Here's how the part is built. I have some questions about the finished solid (model axes, mm). Round coordinates to 2 decimals unless told otherwise and drop trailing zeros. Order: outer loops, then holes, each group sorted by start corner. A loop starts at its lowest first (then second) coordinate and runs counter-clockwise, first axis right, second up. Notation, with made-up numbers: M 22.25,-23 L 44.25,-23 A25 cw 44.25,-11 Z; hole C 16.25,-38 d1. An arc over 180 degrees is marked long. Write item = value, one per line. Start each with the question number.
Item 1: I want a section at C-C, the plane z = -23.5. List the corners of the cut face in (x, y) for me, plus the area to 3 significant figures.
Item 2: I want a section at A-A, the plane x = 23.5. List the corners of the cut face in (y, z) for me, plus the area to 3 significant figures.
Item 3: I want a section at D-D, the plane x = 5. List the corners of the cut face in (y, z) for me, plus the area to 3 significant figures.
Item 4: I want a section at B-B, the plane z = -17.5. List the corners of the cut face in (x, y) for me.
Item 5: Please list where these lines run through material, in increasing order: L1, parallel to Z at x = -23.5, y = 1.1; L2, parallel to X at y = 1.5, z = -23.5; L3, parallel to X at y = 1.55, z = 23.5.
Item 6: I'm going to push flat-ended pins straight in: P1, Ø1, axis at x = 12, y = 0.5, coming from the +Z side; P2, Ø0.6, axis at x = -11.5, y = 1, coming from the -Z side. Where does each tip first touch, or does it pass through?
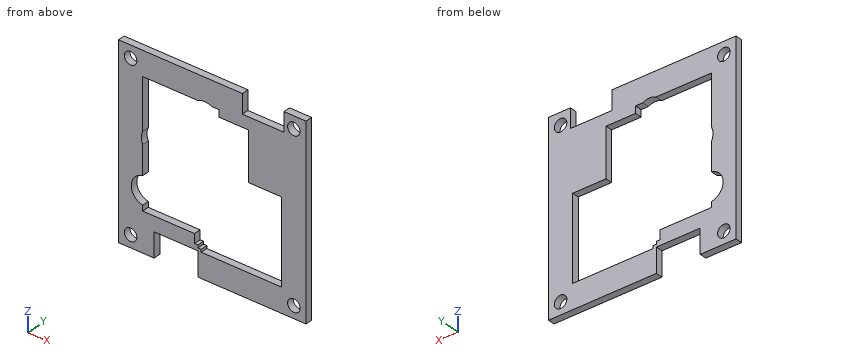
```python
from build123d import *

# Parameters (mm, degrees)
SKETCH_3_R      = 1.8
SKETCH_3_W      = 0.8
SKETCH_3_H      = 1.5
SKETCH_3_W_2    = 1
SKETCH_3_W_3    = 0.944853381
SKETCH_3_H_2    = 0.76832805
EXTRUDE_2_DEPTH = 2


with BuildPart() as part:
    # 草图3 → 凸台-拉伸2 (new body)
    with BuildSketch(Plane(origin=(0, 0, 0), x_dir=(1, 0, 0), z_dir=(0, 1, 0))):
        with BuildLine():
            Line((8.65, -27), (8.65, -21.5))
            Line((8.65, -21.5), (8.65, -20))
            Line((8.65, -20), (1.9, -20))
            Line((1.9, -20), (-0.163508327, -20))
            ThreePointArc((-0.163508327, -20), (-2.1, -20.5), (-4.036491673, -20))
            Line((-4.036491673, -20), (-20, -20))
            Line((-20, -20), (-20, -5.443559577))
            ThreePointArc((-20, -5.443559577), (-20.4, -3.7), (-20, -1.956440423))
            Line((-20, -1.956440423), (-20, 6.361726266))
            ThreePointArc((-20, 6.361726266), (-23.3, 10.3), (-20, 14.238273734))
            Line((-20, 14.238273734), (-20, 15.8))
            Line((-20, 15.8), (-20, 20))
            Line((-20, 20), (-16.7, 20))
            Line((-16.7, 20), (-16.7, 27))
            Line((-16.7, 27), (-27, 27))
            Line((-27, 27), (-27, -27))
            Line((-27, -27), (8.65, -27))
        make_face()
        with Locations((-23.5, -23.5)):
            Circle(SKETCH_3_R, mode=Mode.SUBTRACT)
        with Locations((-23.5, 23.5)):
            Circle(SKETCH_3_R, mode=Mode.SUBTRACT)
        Polygon((20, -18), (20, -20), (20.65, -20), (20.65, -21.5), (20.65, -27), (27, -27), (27, 27), (-4.1, 27), (-4.1, 20), (-3.155146619, 20), (20, 20), (20, -4), align=None)
        with Locations((23.5, -23.5)):
            Circle(SKETCH_3_R, mode=Mode.SUBTRACT)
        with Locations((23.5, 23.5)):
            Circle(SKETCH_3_R, mode=Mode.SUBTRACT)
        Polygon((12.4, -20), (12.4, -19.5), (12.4, -18), (10.4, -18), (1.9, -18), (1.9, -20), (8.65, -20), align=None)
        Polygon((20, -20), (16.9, -20), (16.9, -19.5), (16.1, -19.5), (13.4, -19.5), (12.4, -19.5), (12.4, -20), (8.65, -20), (8.65, -21.5), (20.65, -21.5), (20.65, -20), align=None)
        Polygon((16.9, -19.5), (16.9, -20), (20, -20), (20, -18), (16.9, -18), align=None)
        with Locations((16.5, -18.75)):
            Rectangle(SKETCH_3_W, SKETCH_3_H)
        with Locations((12.9, -18.75)):
            Rectangle(SKETCH_3_W_2, SKETCH_3_H)
        Polygon((16.1, -18), (16.9, -18), (16.9, -6), (12.4, -6), (12.4, -18), (13.4, -18), (13.4, -19.5), (16.1, -19.5), align=None)
        Polygon((16.9, -18), (20, -18), (20, -4), (10.4, -4), (10.4, -6), (10.4, -18), (12.4, -18), (12.4, -6), (16.9, -6), align=None)
        with Locations((-3.62757331, 19.615835975)):
            Rectangle(SKETCH_3_W_3, SKETCH_3_H_2)
        Polygon((-4.1, 19.23167195), (-4.1, 20), (-10.4, 20), (-16.7, 20), (-20, 20), (-20, 15.8), (-5.1, 15.8), (-5.1, 18.463343901), (-4.1, 18.463343901), align=None)
    extrude(amount=EXTRUDE_2_DEPTH)


solid = part.part
```
Filled in:
q1.outline = M -27,0 L -25.3,0 L -25.3,2 L -27,2 Z; M -21.7,0 L -16.7,0 L -16.7,2 L -21.7,2 Z; M -4.1,0 L 21.7,0 L 21.7,2 L -4.1,2 Z; M 25.3,0 L 27,0 L 27,2 L 25.3,2 Z
q1.area = 68.4 mm^2
q2.outline = M 0,-27 L 2,-27 L 2,-25.3 L 0,-25.3 Z; M 0,-21.7 L 2,-21.7 L 2,21.7 L 0,21.7 Z; M 0,25.3 L 2,25.3 L 2,27 L 0,27 Z
q2.area = 93.6 mm^2
q3.outline = M 0,-27 L 2,-27 L 2,-20 L 0,-20 Z; M 0,18 L 2,18 L 2,27 L 0,27 Z
q3.area = 32.0 mm^2
q4.outline = M -27,0 L -5.1,0 L -5.1,2 L -27,2 Z; M 20,0 L 27,0 L 27,2 L 20,2 Z
q5.L1 = -27 to -25.3, -21.7 to 21.7, 25.3 to 27
q5.L2 = -27 to -25.3, -21.7 to -16.7, -4.1 to 21.7, 25.3 to 27
q5.L3 = -27 to -25.3, -21.7 to 8.65, 20.65 to 21.7, 25.3 to 27
q6.P1 = 21.5
q6.P2 = -20
